from build123d import *

# Parameters (mm, degrees)
SKETCH3_R                = 35
SKETCH3_R_2              = 30
BOSS_EXTRUDE1_DEPTH      = 50
BOSS_EXTRUDE2_START      = -5
SKETCH4_R                = 30
BOSS_EXTRUDE2_DEPTH      = 5
REVOLVE1_ANGLE           = 90
SKETCH8_R                = 30
CUT_EXTRUDE2_DEPTH       = 5
BOSS_EXTRUDE4_REACH      = 100.362
BOSS_EXTRUDE4_END_RADIUS = 30
BOSS_EXTRUDE5_REACH      = 100.362
BOSS_EXTRUDE18_DEPTH     = 35
SKETCH13_W               = 35
SKETCH13_H               = 5
BOSS_EXTRUDE19_DEPTH     = 50
BOSS_EXTRUDE20_REACH     = 114.583
SKETCH14_W               = 50
SKETCH14_H               = 5
CUT_EXTRUDE4_START       = -25
SKETCH15_R               = 30
CUT_EXTRUDE4_DEPTH       = 25
CUT_EXTRUDE6_DEPTH       = 116.542200083
CUT_EXTRUDE6_DEPTH_BACK  = 40
BOSS_EXTRUDE21_START     = -32
BOSS_EXTRUDE21_DEPTH     = 32
SKETCH20_W               = 6.358964111
SKETCH20_H               = 20
SKETCH20_W_2             = 46
SKETCH20_W_3             = 5
CUT_EXTRUDE7_DEPTH       = 14


# Read off the part's stored shape, not the designer's step: Shell1
with BuildPart() as part:
    # Sketch3 → Boss-Extrude1 (new body)
    with BuildSketch(Plane(origin=(0, 0, 0), x_dir=(0, 0, -1), z_dir=(1, 0, 0))):
        Circle(SKETCH3_R)
        Circle(SKETCH3_R_2, mode=Mode.SUBTRACT)
    extrude(amount=BOSS_EXTRUDE1_DEPTH)

    # Sketch4 → Boss-Extrude2 (add)
    with BuildSketch(Plane(origin=(50, 0, 0), x_dir=(0, 0, -1), z_dir=(1, 0, 0)).offset(BOSS_EXTRUDE2_START)):
        Circle(SKETCH4_R)
    extrude(amount=BOSS_EXTRUDE2_DEPTH)

    # Sketch5 → Revolve1 (revolve)
    with BuildSketch(Plane(origin=(50, 0, 0), x_dir=(0, 0, -1), z_dir=(1, 0, 0))):
        with BuildLine():
            Line((0, -35), (0, 35))
            ThreePointArc((0, 35), (35, 0), (0, -35))
        make_face()
    revolve(axis=Axis((50, -35, 0), (0, -1, 0)), revolution_arc=REVOLVE1_ANGLE)

    # Shell1 outline → Shell1 (revolve, cut)
    with BuildSketch(Plane.YX):
        with BuildLine():
            Line((0, 80), (0, 50))
            Line((0, 50), (30, 50))
            ThreePointArc((30, 50), (21.213203436, 71.213203436), (0, 80))
        make_face()
    revolve(axis=Axis((0, 0, 0), (1, 0, 0)), mode=Mode.SUBTRACT)

    # Sketch8 → Cut-Extrude2 (cut)
    with BuildSketch(Plane.ZY.offset(-45)):
        with Locations(Location((0, 0, 0), (0, 0, 90))):
            Circle(SKETCH8_R)
    extrude(amount=-CUT_EXTRUDE2_DEPTH, mode=Mode.SUBTRACT)

    # Boss-Extrude4: up to this sphere (the profile starts inside it)
    boss_extrude4_end = Location((50, 0, 0)) * Sphere(BOSS_EXTRUDE4_END_RADIUS, mode=Mode.PRIVATE)
    # Sketch7 → Boss-Extrude4 (add, up to the surface)
    with BuildSketch(Plane.XY, mode=Mode.PRIVATE) as boss_extrude4_sk1:
        Polygon((65.435214922, 10), (65.435214922, 0), (65.435214922, -10), (78.284271247, -10), (78.284271247, 10), align=None)
    boss_extrude4_tool1 = extrude(boss_extrude4_sk1.sketch, amount=-BOSS_EXTRUDE4_REACH, mode=Mode.PRIVATE) & boss_extrude4_end
    add(boss_extrude4_tool1.solids().sort_by_distance((71.859743, 0, 0))[0])

    # Sketch10 → Boss-Extrude5 (add, up to next)
    with BuildSketch(Plane.XY, mode=Mode.PRIVATE) as boss_extrude5_sk1:
        with BuildLine():
            ThreePointArc((50, 35), (15, 0), (50, -35))
            Line((50, -35), (50, -30))
            ThreePointArc((50, -30), (20, 0), (50, 30))
            Line((50, 30), (50, 35))
        make_face()
    boss_extrude5_tool1 = extrude(boss_extrude5_sk1.sketch, amount=BOSS_EXTRUDE5_REACH, mode=Mode.PRIVATE) - part.part
    add(boss_extrude5_tool1.solids().sort_by_distance((49.217376, 32.5, 0))[0])

    # Sketch12 → Boss-Extrude18 (add)
    with BuildSketch(Plane.XY):
        with BuildLine():
            ThreePointArc((78.284271247, 10), (80, 0), (78.284271247, -10))
            ThreePointArc((78.284271247, -10), (67.320508076, -24.494897428), (50, -30))
            Line((50, -30), (50, -35))
            ThreePointArc((50, -35), (85, 0), (50, 35))
            Line((50, 35), (50, 30))
            ThreePointArc((50, 30), (67.320508076, 24.494897428), (78.284271247, 10))
        make_face()
    extrude(amount=BOSS_EXTRUDE18_DEPTH)

    # Sketch13 → Boss-Extrude19 (add)
    with BuildSketch(Plane.ZY.offset(-50)):
        with Locations((17.5, -32.5)):
            Rectangle(SKETCH13_W, SKETCH13_H)
        with Locations((17.5, 32.5)):
            Rectangle(SKETCH13_W, SKETCH13_H)
    extrude(amount=BOSS_EXTRUDE19_DEPTH)

    # Boss-Extrude20: up to this face of the body (flat: up to its plane)
    boss_extrude20_end = Plane(part.part.faces().sort_by_distance((25, 30, 26.513878189))[0])
    # Sketch14 → Boss-Extrude20 (add, up to the picked face)
    with BuildSketch(Plane(origin=(0, -30, 0), x_dir=(1, 0, 0), z_dir=(0, 1, 0)), mode=Mode.PRIVATE) as boss_extrude20_sk1:
        with Locations((25, -32.5)):
            Rectangle(SKETCH14_W, SKETCH14_H)
    boss_extrude20_tool1 = split(extrude(boss_extrude20_sk1.sketch, amount=BOSS_EXTRUDE20_REACH, mode=Mode.PRIVATE), bisect_by=boss_extrude20_end, keep=Keep.BOTH, mode=Mode.PRIVATE)
    add(boss_extrude20_tool1.solids().sort_by(Axis((25, -30, 32.5), (0, 1, 0)))[0])

    # Sketch15 → Cut-Extrude4 (cut)
    with BuildSketch(Plane.XY.offset(35).offset(CUT_EXTRUDE4_START)):
        with Locations(Location((50, 0, 0), (0, 0, 109.471220634))):
            Circle(SKETCH15_R)
    extrude(amount=CUT_EXTRUDE4_DEPTH, mode=Mode.SUBTRACT)

    # Sketch16 → Cut-Extrude6 (cut, two sides: drawn at the far end of the back side and taken through both)
    with BuildSketch(Plane.XY.offset(35).offset(-CUT_EXTRUDE6_DEPTH_BACK)):
        with BuildLine():
            Line((21.715728753, 10), (20, 10))
            Line((20, 10), (20, 0))
            ThreePointArc((20, 0), (20.43204321, 5.073059362), (21.715728753, 10))
        make_face()
        with BuildLine():
            ThreePointArc((21.715728753, -10), (20.43204321, -5.073059362), (20, 0))
            Line((20, 0), (20, -10))
            Line((20, -10), (21.715728753, -10))
        make_face()
    extrude(amount=CUT_EXTRUDE6_DEPTH + CUT_EXTRUDE6_DEPTH_BACK, mode=Mode.SUBTRACT)

    # Sketch16<17> → Boss-Extrude21 (add)
    with BuildSketch(Plane.XY.offset(35).offset(BOSS_EXTRUDE21_START)):
        with BuildLine():
            ThreePointArc((24.019237886, 15), (22.752551286, 12.552949398), (21.715728753, 10))
            Line((21.715728753, 10), (66, 10))
            Line((66, 10), (66, -10))
            Line((66, -10), (21.715728753, -10))
            ThreePointArc((21.715728753, -10), (22.752551286, -12.552949398), (24.019237886, -15))
            Line((24.019237886, -15), (71, -15))
            Line((71, -15), (71, 15))
            Line((71, 15), (24.019237886, 15))
        make_face()
    extrude(amount=BOSS_EXTRUDE21_DEPTH)

    # Sketch20 → Cut-Extrude7 (cut)
    with BuildSketch(Plane.XY.offset(35)):
        with Locations((16.820517945, 0)):
            Rectangle(SKETCH20_W, SKETCH20_H)
        with Locations((43, 0)):
            Rectangle(SKETCH20_W_2, SKETCH20_H)
        with Locations((68.5, 0)):
            Rectangle(SKETCH20_W_3, SKETCH20_H)
    extrude(amount=-CUT_EXTRUDE7_DEPTH, mode=Mode.SUBTRACT)


solid = part.part
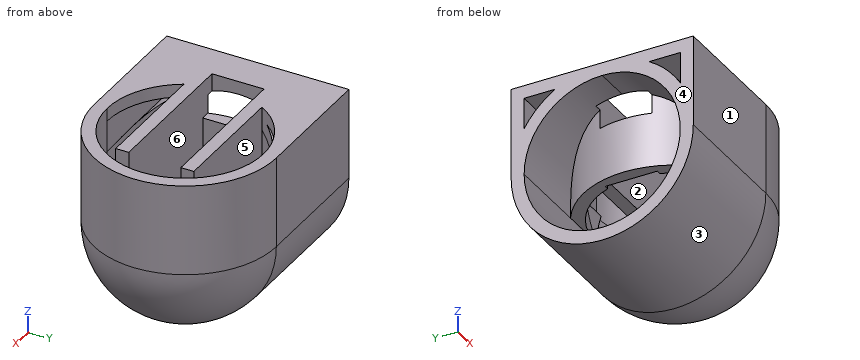
Design review of the part built by this model. Coordinates are the model's own, in mm. Face numbers are marked on the shaded views. A direction names the side the tool comes from. Give positions to 0.01 mm unless a question says otherwise; leave off trailing zeros. Loops run counter-clockwise (first coordinate to the right, second up) from the corner with the lowest first, then second, coordinate; pieces in that order, holes last. Notation, with made-up numbers: M 86,-19.75 L 101,-19.75 A20 ccw 101,-4.75 Z; hole C 82,2 d4. An arc over 180 degrees is marked long. One line per question, with ' | ' between items. Start each with the question number.
1. To check wall thickness, follow L1, parallel to Y at x = 13.5, z = 22.5; L2, parallel to Y at x = 13.5, z = -0.5; L3, parallel to Y at x = 56, z = 28. State the ranges of each line that lie inside material, in increasing order.
2. For the marked faces 1 and 2, list the 3-axis set-ups (+Z, -Z, +X, -X, +Y, -Y) from which the entire face can be reached by the end or side of a thin tool; tool diameter is ignored.
3. Insertion check: P1, Ø2, axis at x = 74, y = 10, coming from the -Z side; P2, Ø3, axis at y = 17, z = 18, coming from the -X side; P3, Ø15, axis at x = 41, y = 2.5, coming from the -Z side. Each pin has a flat end and moves straight along its axis. Give the tip position at first contact, or say it passes through.
4. Add section C-C (y = 5). Write out the cut boundary in (x, z).
5. The part is to be moulded in two halves that separate along Y. For the marked faces 3, 4, 5 and 6, say which applies: released by +Y, released by -Y, zero draft, split by the parting line, or undercut.
6. Add section D-D (x = 37). Write out the cut boundary in (y, z).
7. Add section A-A (x = 9.5). Write out the cut boundary in (y, z), plus the area to 3 significant figures.
8. Add section B-B (z = 24). Write out the cut boundary in (x, y), plus the area to 3 significant figures.
Worked out:
1) L1: y = -35 to -30, -26.81 to -19.84, 19.84 to 26.81, 30 to 35 | L2: y = -35 to -30, 30 to 35 | L3: y = -34.48 to -29.39, -15 to -10, 10 to 15, 29.39 to 34.48
2) face 1: +Z, -Z, +X, -X, -Y | face 2: +Z
3) P1: stops at z = -24.49 | P2: stops at x = 18.62 | P3: stops at z = -35
4) outline: M 0,-34.64 L 50,-34.64 A34.64 ccw 84.64,0 L 84.64,35 L 79.58,35 L 79.58,0 A29.58 cw 78.28,-8.66 L 78.28,0 L 65.44,0 L 65.44,-25.23 A29.58 cw 50,-29.58 L 0,-29.58 Z; M 0,29.58 L 13.64,29.58 L 13.64,35 L 0,35 Z; M 15.36,0 L 20,0 L 20,21 L 15.36,21 Z; M 66,3 L 71,3 L 71,21 L 66,21 Z
5) face 3: split by the parting line | face 4: zero draft | face 5: undercut | face 6: undercut
6) outline: M -35,0 A35 ccw 35,0 L 35,35 L 27.04,35 L 27.04,30 L 30,30 L 30,18.03 A35 ccw 27.04,22.23 L 27.04,0 L 30,0 A30 cw -30,0 L -27.04,0 L -27.04,22.23 A35 ccw -30,18.03 L -30,30 L -27.04,30 L -27.04,35 L -35,35 Z; M -15,3 L -10,3 L -10,35 L -15,35 Z; M 10,3 L 15,3 L 15,35 L 10,35 Z
7) outline: M -35,0 A35 ccw 35,0 L 35,35 L -35,35 Z; hole C 0,0 d60; hole M -30,18.03 A35 cw -18.03,30 L -30,30 Z; hole M 18.03,30 A35 cw 30,18.03 L 30,30 Z | area: 1,430 mm²
8) outline: M 0,-35 L 50,-35 A35 ccw 50,35 L 0,35 L 0,30 L 50,30 A30 cw 50,-30 L 0,-30 Z; M 0,-25.48 L 34.16,-25.48 A30 cw 24.02,-15 L 71,-15 L 71,-10 L 16.46,-10 A35 ccw 19.98,-18 L 0,-18 Z; M 0,18 L 19.98,18 A35 ccw 16.46,10 L 71,10 L 71,15 L 24.02,15 A30 cw 34.16,25.48 L 0,25.48 Z | area: 2,020 mm²
